from build123d import *

# Parameters (mm, degrees)
F0_R          = 9.398
F1_DEPTH      = 13.97
F1_DEPTH_BACK = 13.97
F4_D          = 6.7564
F5_W          = 11.43
F5_H          = 25.3408506978
F6_DEPTH      = 2.54
F7_R          = 0.508


with BuildPart() as f1:
    # F0 (on Front) → F1 (new body, two sides)
    with BuildSketch(Plane.XZ) as f1_sk:
        Circle(F0_R)
    extrude(amount=F1_DEPTH)
    extrude(f1_sk.sketch, amount=-F1_DEPTH_BACK)

    # F4 (through all)
    with Locations(Plane.YZ.offset(10.033)):
        with Locations((0, 0)):
            Hole(F4_D / 2)

    # F5 (on offset) → F6 (cut)
    with BuildSketch(Plane.YZ.offset(10.033)):
        Rectangle(F5_W, F5_H)
    extrude(amount=-F6_DEPTH, mode=Mode.SUBTRACT)

    # F7
    f7_edges = [f1.edges().sort_by_distance(p)[0] for p in [
        (-9.398, 13.97, 0),
        (-9.398, -13.97, 0),
        (8.90903, 5.715, 2.991922),
        (8.90903, 5.715, -2.991922),
        (8.90903, -5.715, 2.991922),
        (8.90903, -5.715, -2.991922),
    ]]
    fillet(f7_edges, radius=F7_R)


solid = f1.part
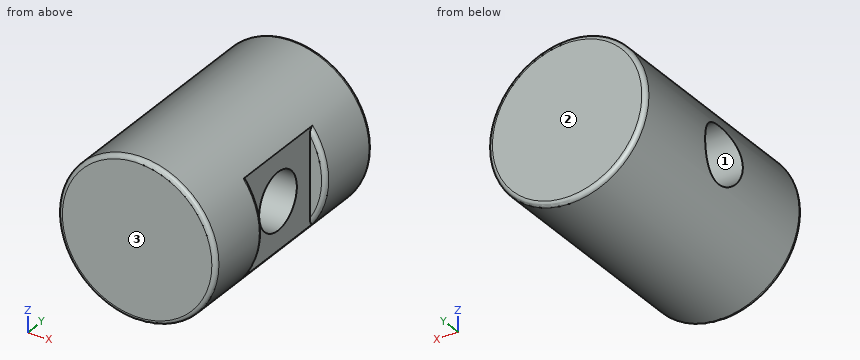
Part model, mm, in its own coordinate system. Face numbers are marked on the shaded views. Coordinates: 2 decimals unless noted, no trailing zeros. Order: outer loops, then holes, each group sorted by start corner. A loop starts at its lowest first (then second) coordinate and runs counter-clockwise, first axis right, second up.
(1) Slice it at D-D, the plane y = -2.5. Write the cut outline in (x, z), and give its area (3 significant figures).
Check sheet entries:
outline: (-9.12, -2.27) arc R9.4 ccw to (7.49, -5.67) - (7.49, -2.27) - close; (-9.12, 2.27) - (7.49, 2.27) - (7.49, 5.67) arc R9.4 ccw to start
area: 186 mm2
(2) Slice it at B-B, the plane z = 0. Write the cut outline in (x, y) (3 decimals).
Check sheet entries:
outline: (-9.398, -13.462) arc R0.508 ccw to (-8.89, -13.97) - (8.89, -13.97) arc R0.508 ccw to (9.398, -13.462) - (9.398, -6.223) arc R0.508 ccw to (8.89, -5.715) - (7.493, -5.715) - (7.493, -3.378) - (-9.398, -3.378) - close; (-9.398, 3.378) - (7.493, 3.378) - (7.493, 5.715) - (8.89, 5.715) arc R0.508 ccw to (9.398, 6.223) - (9.398, 13.462) arc R0.508 ccw to (8.89, 13.97) - (-8.89, 13.97) arc R0.508 ccw to (-9.398, 13.462) - close
(3) Slice it at A-A, the plane x = 0. Write the cut outline in (y, z), and give its area (3 significant figures).
Check sheet entries:
outline: (-13.97, -8.89) arc R0.51 ccw to (-13.46, -9.4) - (13.46, -9.4) arc R0.51 ccw to (13.97, -8.89) - (13.97, 8.89) arc R0.51 ccw to (13.46, 9.4) - (-13.46, 9.4) arc R0.51 ccw to (-13.97, 8.89) - close; hole circle Ø6.76 at (0, 0)
area: 489 mm2
(4) Probe L1, parallel to Y at x = -5, z = 0; L2, parallel to Z at x = -0.75, y = -2; L3, parallel to Z at x = -3.5, y = 0. List the from-to ranges inside material, lowest first.
Check sheet entries:
L1: y = -13.97 to -3.38, 3.38 to 13.97
L2: z = -9.37 to -2.72, 2.72 to 9.37
L3: z = -8.72 to -3.38, 3.38 to 8.72
(5) Pull direction Y, two halves, no side cores. Call the marked faces 1, 2 and 3: pulls with the +Y half, pulls with the -Y half, needs draft (parallel to the pull), parting line crosses it, or undercut.
Check sheet entries:
face 1: undercut
face 2: pulls with the +Y half
face 3: pulls with the -Y half
(6) Slice it at C-C, the plane y = 2.25. Write the cut outline in (x, z), and give its area (3 significant figures).
Check sheet entries:
outline: (-9.05, -2.52) arc R9.4 ccw to (7.49, -5.67) - (7.49, -2.52) - close; (-9.05, 2.52) - (7.49, 2.52) - (7.49, 5.67) arc R9.4 ccw to start
area: 178 mm2
(7) Pin check, flat tips, straight feed: pin 1 Ø2 at (y, z) = (-10.5, 7) entering from -X; pin 2 Ø2 at (y, z) = (-8.5, 3.5) entering from -X; pin 3 Ø9 at (y, z) = (0, 0) entering from +X. Stop position of each tip, or through.
Check sheet entries:
pin 1: stops at x = -7.23
pin 2: stops at x = -9.06
pin 3: stops at x = 7.49
